The figure shows three views and two pictorial views of one solid part (mm, origin at its lowest corner). Answer the questions. A direction names the side the tool comes from. Give positions to 0.01 mm unless a question says otherwise; leave off trailing zeros. Loops run counter-clockwise (first coordinate to the right, second up) from the corner with the lowest first, then second, coordinate; pieces in that order, holes last. Notation, with made-up numbers: (54, -9) - (79, -9) arc R29 cw to (79, 15) - close; hole circle Ø5 at (-21, 73). An arc over 180 degrees is marked (long way). One line per question, with ' | ' between items.
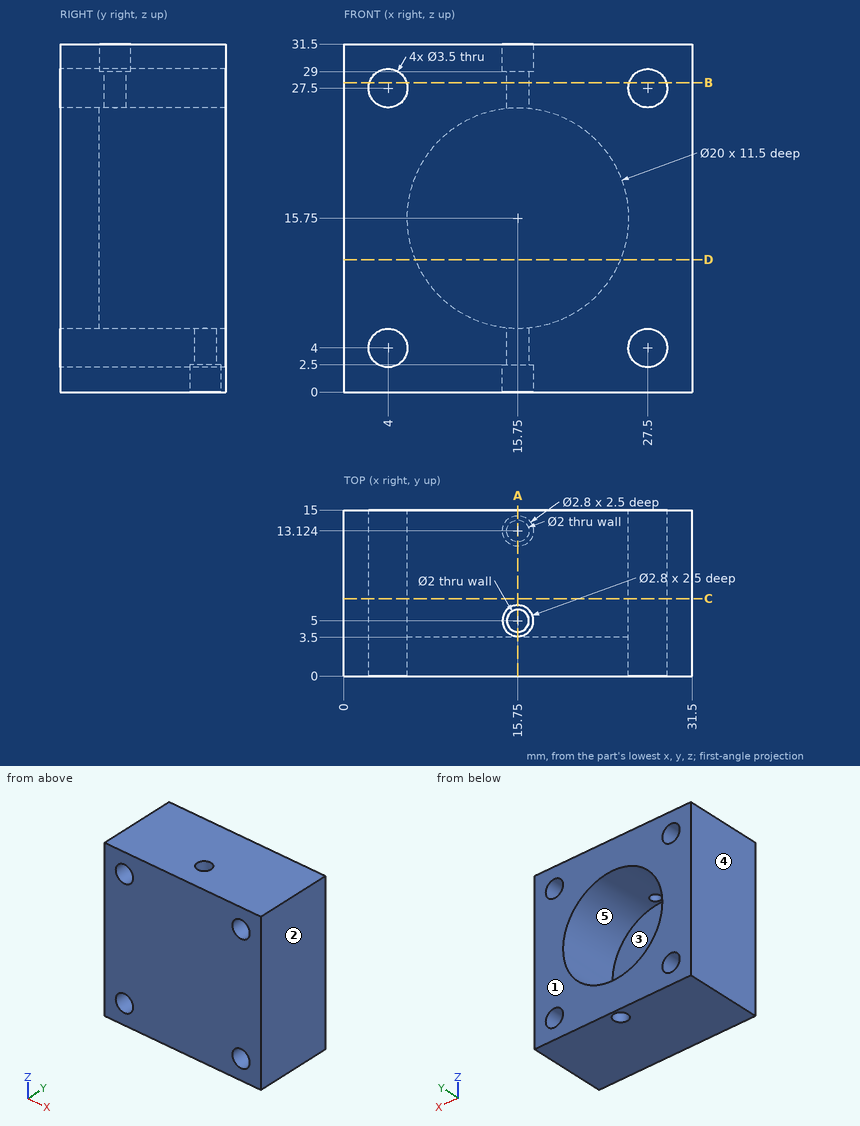
1. Which of the six approach directions +Z, -Z, +X, -X, +Y, -Y give full straight-line access (tool end or side, diameter ignored) to the marked faces 4 and 5?
Evaluation:
face 4: +Z, -Z, -X, +Y, -Y | face 5: +Y
2. Find section B-B on z = 28. Write down the section's boundary in (x, y), then the cut area to 3 significant figures.
Evaluation:
outline: (0, 0) - (2.32, 0) - (2.32, 15) - (0, 15) - close; (5.68, 0) - (25.82, 0) - (25.82, 15) - (5.68, 15) - close; (29.18, 0) - (31.5, 0) - (31.5, 15) - (29.18, 15) - close; hole circle Ø2 at (15.75, 5) | area: 369 mm2
3. Determine the mould class of the marked faces 1, 2 and 3 for opening direction X: +X half, -X half, draft (parallel to the pull), parting line (faces both ways), or undercut.
Evaluation:
face 1: draft | face 2: +X half | face 3: undercut
4. Find section D-D on z = 12. Write down the section's boundary in (x, y).
Evaluation:
outline: (0, 0) - (31.5, 0) - (31.5, 15) - (25.02, 15) - (25.02, 3.5) - (6.48, 3.5) - (6.48, 15) - (0, 15) - close
5. Consider L1, parallel to X at y = 6.25, z = 4; L2, parallel to Z at x = 15.75, y = 8.75; L3, parallel to Z at x = 3, y = 9.75 (1 decimal). Determine where each line is inside the solid, lowest interval first.
Evaluation:
L1: 0 to 2.25, 5.75 to 25.75, 29.25 to 31.5 | L2: 0 to 5.75, 25.75 to 31.5 | L3: 0 to 2.6, 5.4 to 26.1, 28.9 to 31.5
6. Find section A-A on x = 15.75. Write down the section's boundary in (y, z).
Evaluation:
outline: (0, 0) - (11.72, 0) - (11.72, 2.5) - (12.12, 2.5) - (12.12, 5.75) - (3.5, 5.75) - (3.5, 25.75) - (4, 25.75) - (4, 29) - (3.6, 29) - (3.6, 31.5) - (0, 31.5) - close; (6, 25.75) - (15, 25.75) - (15, 31.5) - (6.4, 31.5) - (6.4, 29) - (6, 29) - close; (14.12, 2.5) - (14.52, 2.5) - (14.52, 0) - (15, 0) - (15, 5.75) - (14.12, 5.75) - close
7. Find section C-C on y = 7. Write down the section's boundary in (x, z).
Evaluation:
outline: (0, 0) - (31.5, 0) - (31.5, 31.5) - (0, 31.5) - close; hole circle Ø3.5 at (4, 4); hole circle Ø3.5 at (4, 27.5); hole circle Ø20 at (15.75, 15.75); hole circle Ø3.5 at (27.5, 4); hole circle Ø3.5 at (27.5, 27.5)
8. Flat-ended cylindrical pins translate along their axes: pin 1 (2 mm diameter, centred on x = 4, z = 4, fed in from -Y); pin 2 (1 mm diameter, centred on x = 13.5, z = 18.5, fed in from +Y); pin 3 (1.4 mm diameter, centred on x = 15.5, y = 13.5, fed in from -Z). Find the tip coordinate at first contact, or state that the pin passes through.
Evaluation:
pin 1: through | pin 2: y = 3.5 | pin 3: z = 2.5
